Could you check a few things on this model? Use its own coordinates, in mm. Face numbers are marked on the shaded views. A direction names the side the tool comes from. Give positions to 0.01 mm unless a question says otherwise; leave off trailing zeros. Loops run counter-clockwise (first coordinate to the right, second up) from the corner with the lowest first, then second, coordinate; pieces in that order, holes last. Notation, with made-up numbers: (61, 25) - (93, 25) arc R20 ccw to (93, 64) - close; hole circle Ø1 at (19.5, 85.5). An arc over 180 degrees is marked (long way). Write each question's results on one line, items separated by ' | '. Start each with the question number.
1) I want a section at C-C, the plane z = -18.5. Count the separate pieces of the cut face and the enclosed holes in it, and give its area (3 significant figures).
2) I'm going to push flat-ended pins straight in: pin 1 (3.5 mm diameter, centred on x = -0.5, z = -8.5, fed in from +Y); pin 2 (3.5 mm diameter, centred on x = -2.5, z = 0, fed in from -Y); pin 3 (4 mm diameter, centred on y = -14, z = 16.5, fed in from +X). Where does each tip first touch, or does it pass through?
3) If I drill on probe 1 along X at (y, z) = (22, 20); probe 2 along X at (y, z) = (18, 13); probe 3 along X at (y, z) = (12.5, 14), over which ranges is the centre line in solid material (lowest first)? Write a range as [from, to].
4) If we mould it in two halves opening along X, with no side actions, what happens to the marked faces 1, 2, 3 and 4? For each: +X half, -X half, draft (parallel to the pull), parting line (faces both ways), or undercut.
5) I want a section at A-A, the plane y = 0. Write out the boundary of the cut face in (x, z), and give its area (3 significant figures).
6) On a 3-axis mill with a long thin cutter (end or side, diameter ignored), from which of +Z, -Z, +X, -X, +Y, -Y can I reach the whole of each face in a straight line? I mean the marked faces 5, 6 and 7. Say none if no direction works.
7) I want a section at B-B, the plane x = -31. Write out the boundary of the cut face in (y, z), and give its area (3 significant figures).
8) I want a section at D-D, the plane x = -8. Write out the boundary of the cut face in (y, z), and give its area (3 significant figures).
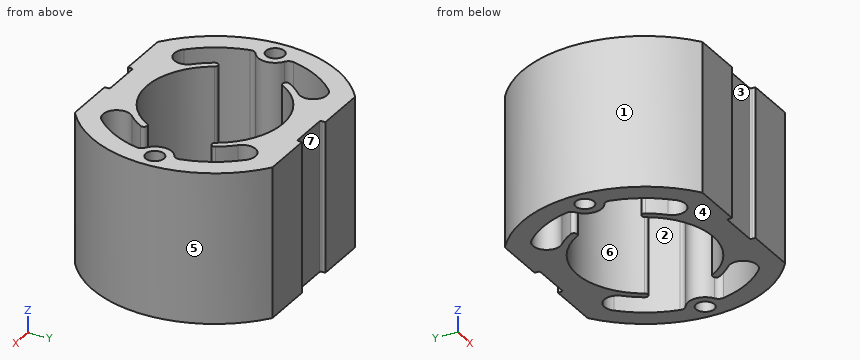
from build123d import *

# Parameters (mm, degrees)
ESQUISSE1_R      = 2.7
EXTRUSION1_DEPTH = 22


with BuildPart() as part:
    # Esquisse1 → Extrusion1 (new, symmetric)
    with BuildSketch(Plane.XY):
        with BuildLine():
            Line((-21.330729008, 29), (-6, 29))
            Line((-6, 29), (-6, 28))
            ThreePointArc((-6, 28), (-5.853553391, 27.646446609), (-5.5, 27.5))
            Line((-5.5, 27.5), (5.5, 27.5))
            ThreePointArc((5.5, 27.5), (5.853553391, 27.646446609), (6, 28))
            Line((6, 28), (6, 29))
            Line((6, 29), (21.330729008, 29))
            ThreePointArc((21.330729008, 29), (36, 0), (21.330729008, -29))
            Line((21.330729008, -29), (6, -29))
            Line((6, -29), (6, -28))
            ThreePointArc((6, -28), (5.853553391, -27.646446609), (5.5, -27.5))
            Line((5.5, -27.5), (-5.5, -27.5))
            ThreePointArc((-5.5, -27.5), (-5.853553391, -27.646446609), (-6, -28))
            Line((-6, -28), (-6, -29))
            Line((-6, -29), (-21.330729008, -29))
            ThreePointArc((-21.330729008, -29), (-36, 0), (-21.330729008, 29))
        make_face()
        with Locations((-31, 0)):
            Circle(ESQUISSE1_R, mode=Mode.SUBTRACT)
        with Locations(Location((31, 0, 0), (0, 0, 180))):
            Circle(ESQUISSE1_R, mode=Mode.SUBTRACT)
        with BuildLine():
            ThreePointArc((-17.320508076, 10), (-18.686533479, 9.633974596), (-19.052558883, 11))
            ThreePointArc((-19.052558883, 11), (-17.453773486, 13.392751438), (-15.556349186, 15.556349186))
            ThreePointArc((-15.556349186, 15.556349186), (-15.556349186, 21.213203436), (-21.213203436, 21.213203436))
            ThreePointArc((-21.213203436, 21.213203436), (-26.32401055, 14.389109374), (-29.30875576, 6.402877149))
            ThreePointArc((-29.30875576, 6.402877149), (-29.193831331, 5.189821407), (-28.396313364, 4.268584766))
            ThreePointArc((-28.396313364, 4.268584766), (-26, 0), (-28.396313364, -4.268584766))
            ThreePointArc((-28.396313364, -4.268584766), (-29.193831331, -5.189821407), (-29.30875576, -6.402877149))
            ThreePointArc((-29.30875576, -6.402877149), (-26.32401055, -14.389109374), (-21.213203436, -21.213203436))
            ThreePointArc((-21.213203436, -21.213203436), (-15.556349186, -21.213203436), (-15.556349186, -15.556349186))
            ThreePointArc((-15.556349186, -15.556349186), (-17.453773486, -13.392751438), (-19.052558883, -11))
            ThreePointArc((-19.052558883, -11), (-18.686533479, -9.633974596), (-17.320508076, -10))
            ThreePointArc((-17.320508076, -10), (0, -20), (17.320508076, -10))
            ThreePointArc((17.320508076, -10), (18.686533479, -9.633974596), (19.052558883, -11))
            ThreePointArc((19.052558883, -11), (17.453773486, -13.392751438), (15.556349186, -15.556349186))
            ThreePointArc((15.556349186, -15.556349186), (15.556349186, -21.213203436), (21.213203436, -21.213203436))
            ThreePointArc((21.213203436, -21.213203436), (26.32401055, -14.389109374), (29.30875576, -6.402877149))
            ThreePointArc((29.30875576, -6.402877149), (29.193831331, -5.189821407), (28.396313364, -4.268584766))
            ThreePointArc((28.396313364, -4.268584766), (26, 0), (28.396313364, 4.268584766))
            ThreePointArc((28.396313364, 4.268584766), (29.193831331, 5.189821407), (29.30875576, 6.402877149))
            ThreePointArc((29.30875576, 6.402877149), (26.32401055, 14.389109374), (21.213203436, 21.213203436))
            ThreePointArc((21.213203436, 21.213203436), (15.556349186, 21.213203436), (15.556349186, 15.556349186))
            ThreePointArc((15.556349186, 15.556349186), (17.453773486, 13.392751438), (19.052558883, 11))
            ThreePointArc((19.052558883, 11), (18.686533479, 9.633974596), (17.320508076, 10))
            ThreePointArc((17.320508076, 10), (0, 20), (-17.320508076, 10))
        make_face(mode=Mode.SUBTRACT)
    extrude(amount=EXTRUSION1_DEPTH, both=True)


solid = part.part
Answers:
1) separate pieces: 1 | enclosed holes: 3 | area: 1,550 mm2
2) pin 1: stops at y = 27.5 | pin 2: stops at y = -27.5 | pin 3: stops at x = 33.94
3) probe 1: x = [-28.5, -20.1], [-16.67, 16.67], [20.1, 28.5] | probe 2: x = [-31.18, -24], [-14.4, -8.72], [8.72, 14.4], [24, 31.18] | probe 3: x = [-33.76, -27.27], [-18.1, -15.61], [15.61, 18.1], [27.27, 33.76]
4) face 1: -X half | face 2: undercut | face 3: undercut | face 4: draft
5) outline: (-36, -22) - (-33.7, -22) - (-33.7, 22) - (-36, 22) - close; (-28.3, -22) - (-26, -22) - (-26, 22) - (-28.3, 22) - close; (26, -22) - (28.3, -22) - (28.3, 22) - (26, 22) - close; (33.7, -22) - (36, -22) - (36, 22) - (33.7, 22) - close | area: 405 mm2
6) face 5: +Z, -Z, +X | face 6: +Z, -Z | face 7: +Z, -Z, +Y
7) outline: (-18.3, -22) - (-2.7, -22) - (-2.7, 22) - (-18.3, 22) - close; (2.7, -22) - (18.3, -22) - (18.3, 22) - (2.7, 22) - close | area: 1,370 mm2
8) outline: (-29, -22) - (-18.33, -22) - (-18.33, 22) - (-29, 22) - close; (18.33, -22) - (29, -22) - (29, 22) - (18.33, 22) - close | area: 939 mm2
